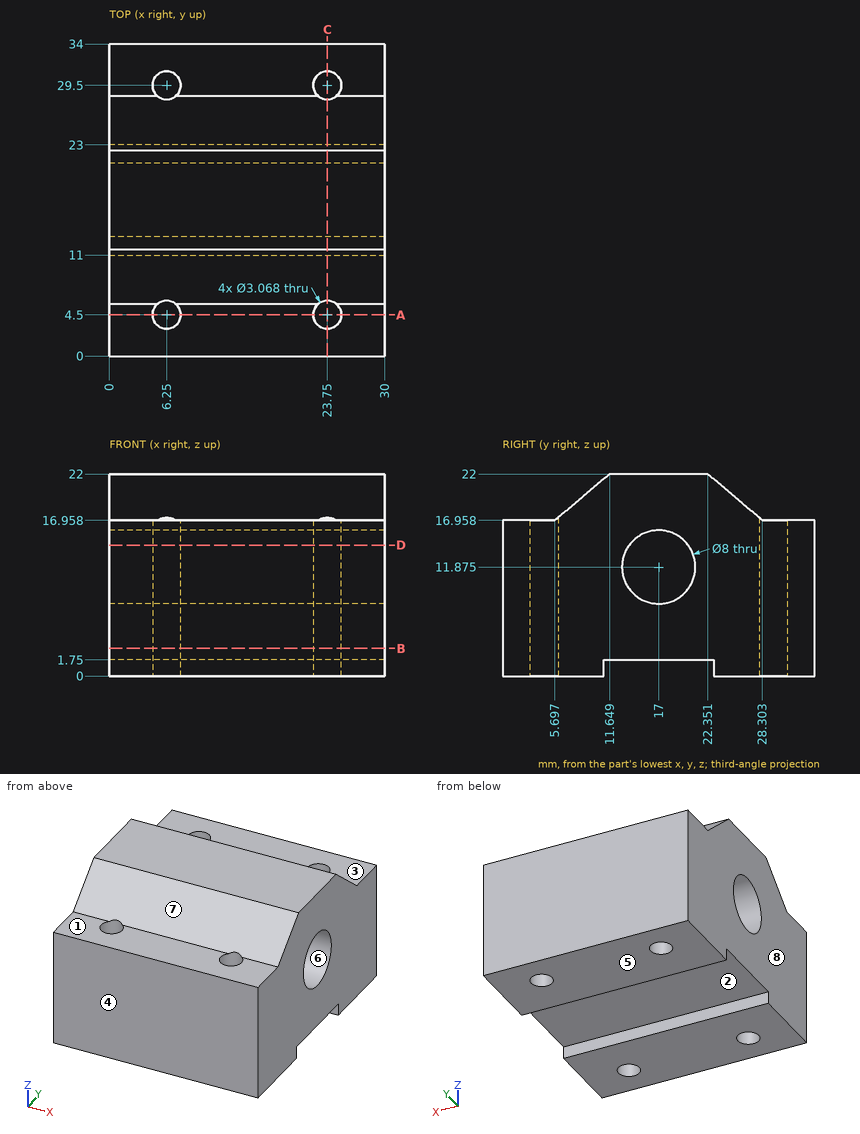
For this review, use the dimensioned drawing (mm, ordinates from the lowest corner) and the shaded views. A direction names the side the tool comes from. Give positions to 0.01 mm unless a question says otherwise; leave off trailing zeros. Write each loop counter-clockwise with the first axis right and the second up, starting at its lowest first coordinate (ties: lowest second). Pieces come first, ordered by that corner, then holes.
(1) Consider section C-C, the plane x = 23.75. Give the number of separate pieces and of enclosed holes in the cut face, and give its area (3 significant figures).
(2) Consider section A-A, the plane y = 4.5. Give the boundary of the cut face in (x, z).
(3) For P1, Ø5, axis at x = 6.25, y = 4.5, coming from the +Z side; P2, Ø4, axis at x = 8.5, y = 4, coming from the +Z side (1 decimal); P3, Ø6.5, axis at x = 14, y = 30.5, coming from the +Z side, all flat-tipped, find the tip position at first contact; note any pin that passes through.
(4) To check wall thickness, follow L1, parallel to Y at x = 6.25, z = 5.5; L2, parallel to Y at x = 6.25, z = 12; L3, parallel to Y at x = 23.75, z = 13.75 (1 decimal). State the ranges of each line that lie inside material, in increasing order.
(5) The part is to be moulded in two halves that separate along Y. For the marked faces 6, 7 and 8, say which applies: released by +Y, released by -Y, zero draft, split by the parting line, or undercut.
(6) Tool access review of the marked faces 1, 2, 3, 4 and 5: name each direction out of +Z, -Z, +X, -X, +Y, -Y from which nothing blocks a thin tool from reaching the whole face with its end or side.
(7) Consider section D-D, the plane z = 14.25. Give the boundary of the cut face in (x, y).
(8) Consider section B-B, the plane z = 3. Give the boundary of the cut face in (x, y).
Returned:
1. separate pieces: 3
1. enclosed holes: 1
1. area: 485 mm2
2. outline: (0, 0) - (4.72, 0) - (4.72, 16.96) - (0, 16.96) - close; (7.78, 0) - (22.22, 0) - (22.22, 16.96) - (7.78, 16.96) - close; (25.28, 0) - (30, 0) - (30, 16.96) - (25.28, 16.96) - close
3. P1: stops at z = 18.06
3. P2: stops at z = 17.2
3. P3: stops at z = 17.85
4. L1: y = 0 to 2.97, 6.03 to 27.97, 31.03 to 34
4. L2: y = 0 to 2.97, 6.03 to 13, 21 to 27.97, 31.03 to 34
4. L3: y = 0 to 3, 6 to 13.5, 20.5 to 28, 31 to 34
5. face 6: undercut
5. face 7: released by -Y
5. face 8: zero draft
6. face 1: +Z, +X, -X, -Y
6. face 2: -Z, +X, -X
6. face 3: +Z, +X, -X, +Y
6. face 4: +Z, -Z, +X, -X, -Y
6. face 5: -Z, +X, -X, +Y, -Y
7. outline: (0, 0) - (30, 0) - (30, 13.78) - (0, 13.78) - close; (0, 20.22) - (30, 20.22) - (30, 34) - (0, 34) - close; hole circle Ø3.07 at (6.25, 4.5); hole circle Ø3.07 at (6.25, 29.5); hole circle Ø3.07 at (23.75, 4.5); hole circle Ø3.07 at (23.75, 29.5)
8. outline: (0, 0) - (30, 0) - (30, 34) - (0, 34) - close; hole circle Ø3.07 at (6.25, 4.5); hole circle Ø3.07 at (6.25, 29.5); hole circle Ø3.07 at (23.75, 4.5); hole circle Ø3.07 at (23.75, 29.5)
